Geometry check sheet. Reference: the model listing, model coordinates, mm. A direction names the side the tool comes from. Give positions to 0.01 mm unless a question says otherwise; leave off trailing zeros. Write each loop counter-clockwise with the first axis right and the second up, starting at its lowest first coordinate (ties: lowest second). Pieces come first, ordered by that corner, then holes.
(1) Cross-section at D-D (z = 1.75). Record the boundary of the cut face in (x, y).
(2) Depth check by flat-ended pin: P1, Ø1.5, axis at y = 31, z = 9.5, coming from the -X side; P2, Ø1.9, axis at x = 4, y = 31, coming from the -Z side; P3, Ø6, axis at x = 12, y = 30.5, coming from the +Z side; P4, Ø10, axis at x = 7.5, z = 12.5, coming from the -Y side. Enter the tip coordinate at first touch or a pass-through.
(3) Mould release check, pull along Y, two halves, no side actions. Record for faces 4 (the flat face through (3, 25, 19.05)), 5 (the flat face through (25, 50.8, 19)), 6 (the flat face through (46, 25, 21.59)): +Y half, -Y half, draft (parallel to the pull), parting line (faces both ways), or undercut.
(4) Cross-section at B-B (z = 17). Record the boundary of the cut face in (x, y).
(5) Cross-section at C-C (x = 16.5). Record the boundary of the cut face in (y, z).
(6) Tool access check on faces 1 (the flat face through (2.54, 25, 23)), 2 (the flat face through (0, 25, 22)), 3 (the flat face through (48, 25, 19.05)). Record the directions out of +Z, -Z, +X, -X, +Y, -Y that give a thin tool (end or side, any length) a straight path to the whole face; none if there is none.
(7) Thickness scan on line 1 along X through (y, z) = (3, 23.5); line 2 along X through (y, z) = (3, 8). Record the ranges inside material, lowest first.
(8) Cross-section at A-A (y = 31). Record the boundary of the cut face in (x, z), and give its area (3 significant figures).
```python
from build123d import *

# Parameters (mm, degrees)
F0_W     = 50.8
F0_H     = 25.4
F1_DEPTH = 50.8
F3_DEPTH = 50.8
F5_DEPTH = 50.8
F6_T     = -2.54


with BuildPart() as f1:
    # F0 (on Front) → F1 (new body)
    with BuildSketch(Plane.XZ):
        with Locations((25.4, 12.7)):
            Rectangle(F0_W, F0_H)
    extrude(amount=-F1_DEPTH)

    # F2 (on face) → F3 (cut)
    with BuildSketch(Plane.XZ):
        Polygon((0, 19.05), (0, 0), (25.4, 0), (6.35, 19.05), align=None)
    extrude(amount=-F3_DEPTH, mode=Mode.SUBTRACT)

    # F4 (on face) → F5 (cut)
    with BuildSketch(Plane.XZ):
        Polygon((25.4, 0), (50.8, 0), (50.8, 19.05), (44.45, 19.05), align=None)
    extrude(amount=-F5_DEPTH, mode=Mode.SUBTRACT)

    # F6
    f6_openings = [f1.faces().sort_by_distance(p)[0] for p in [
        (25.4, 25.4, 25.4),
    ]]
    offset(amount=F6_T, openings=f6_openings, kind=Kind.INTERSECTION)


solid = f1.part
```
Reply:
1. outline: (23.65, 0) - (27.15, 0) - (27.15, 50.8) - (23.65, 50.8) - close
2. P1: stops at x = 15.15
2. P2: stops at z = 19.05
2. P3: stops at z = 19.99
2. P4: stops at y = 0
3. face 4: draft
3. face 5: +Y half
3. face 6: undercut
4. outline: (8.4, 0) - (42.4, 0) - (42.4, 50.8) - (8.4, 50.8) - close; hole (11.99, 2.54) - (38.81, 2.54) - (38.81, 48.26) - (11.99, 48.26) - close
5. outline: (0, 8.9) - (50.8, 8.9) - (50.8, 25.4) - (48.26, 25.4) - (48.26, 12.49) - (2.54, 12.49) - (2.54, 25.4) - (0, 25.4) - close
6. face 1: +Z
6. face 2: +Z, -Z, -X, +Y, -Y
6. face 3: -Z, +X, +Y, -Y
7. line 1: x = 0 to 2.54, 48.26 to 50.8
7. line 2: x = 17.4 to 20.99, 29.81 to 33.4
8. outline: (0, 19.05) - (6.35, 19.05) - (25.4, 0) - (44.45, 19.05) - (50.8, 19.05) - (50.8, 25.4) - (48.26, 25.4) - (48.26, 21.59) - (43.4, 21.59) - (25.4, 3.59) - (7.4, 21.59) - (2.54, 21.59) - (2.54, 25.4) - (0, 25.4) - close
8. area: 187 mm2
